Source: CAD feature listing. Evaluate the final solid. Frame: model axes, mm. Coordinates: 2 decimals unless noted, no trailing zeros. Write item = value, one per line. Start each with the question number.
1. Line query: line 1 along X through (y, z) = (21, -3.65); line 2 along X through (y, z) = (0.5, -3.2); line 3 along Y through (x, z) = (-21, -1.2). Output: solid intervals per line, ascending.
2. Section query A-A (x = 29). Give the number of separate pieces and of enclosed holes in the cut face, then the cut area to 3 significant figures.
3. Pin query (flat end, axial travel): pin 1 Ø1.5 at (x, y) = (9, -19.5) entering from +Z; pin 2 Ø1.5 at (x, z) = (0, -2) entering from -Y; pin 3 Ø1.5 at (y, z) = (-13, -2.5) entering from -X; pin 4 Ø1 at (y, z) = (-14.5, -1.5) entering from +X. Return the tip coordinate at first contact, or that it passes through.
```python
from build123d import *

# Parameters (mm, degrees)
F2_DEPTH = 5.08
F3_DEPTH = 5.08


with BuildPart() as f2:
    # F1 (on Top) → F2 (new body)
    with BuildSketch(Plane.XY):
        with BuildLine():
            add(Edge.make_bspline(
                [(-40.3796768019, 31.486727974), (-25.4125832668, 19.5130531459), (4.2719382832, -4.2719382832), (-19.5130531459, 25.4125832668), (-31.486727974, 40.3796768019)],
                knots=[0, 0, 0, 0, 0.5, 1, 1, 1, 1], degree=3))
            Line((-40.3796768019, 31.486727974), (-43.9717792504, 27.8946255256))
            add(Edge.make_bspline(
                [(-43.9717792504, 27.8946255256), (-39.0223614388, 18.5744758569), (-29.1485977035, -0.0186111101), (-39.1966306531, -18.3497362141), (-44.207889928, -27.4920251734)],
                knots=[0, 0, 0, 0, 0.5012696216, 1, 1, 1, 1], degree=3))
            Line((-44.207889928, -27.4920251734), (-40.688852268, -31.1557355805))
            add(Edge.make_bspline(
                [(-40.688852268, -31.1557355805), (-25.5161789229, -19.5156604784), (3.9712190003, 4.6498080898), (-18.7967685048, -26.1767940312), (-30.6525350904, -41.1896309485)],
                knots=[0, 0, 0, 0, 0.4995827747, 1, 1, 1, 1], degree=3))
            Line((-30.6525350904, -41.1896309485), (-26.9813712251, -44.7008922424))
            add(Edge.make_bspline(
                [(-26.9813712251, -44.7008922424), (-17.9946084514, -39.4329857114), (-0.010494669, -28.8909659837), (18.0580501184, -39.3550908644), (27.0976414843, -44.5902337071)],
                knots=[0, 0, 0, 0, 0.4997056226, 1, 1, 1, 1], degree=3))
            Line((27.0976414843, -44.5902337071), (30.7701121053, -41.0803391876))
            add(Edge.make_bspline(
                [(30.7701121053, -41.0803391876), (18.791953604, -26.107641061), (-4.1552313798, 4.3732948199), (25.8949419877, -19.0260044621), (40.8564309314, -30.995195617)],
                knots=[0, 0, 0, 0, 0.5001872305, 1, 1, 1, 1], degree=3))
            Line((40.8564309314, -30.995195617), (44.3699422534, -27.3261850978))
            add(Edge.make_bspline(
                [(44.5902337071, 27.0976414843), (39.403270189, 18.0788208761), (29.0172364099, 0.0201290891), (39.2483982347, -18.2036660263), (44.3699422534, -27.3261850978)],
                knots=[0, 0, 0, 0, 0.4994171624, 1, 1, 1, 1], degree=3))
            Line((44.5902337071, 27.0976414843), (41.0803391876, 30.7701121053))
            add(Edge.make_bspline(
                [(30.995195617, 40.8564309314), (19.0260044621, 25.8949419877), (-4.3732948199, -4.1552313798), (26.107641061, 18.791953604), (41.0803391876, 30.7701121053)],
                knots=[0, 0, 0, 0, 0.4998127695, 1, 1, 1, 1], degree=3))
            Line((30.995195617, 40.8564309314), (27.3261850978, 44.3699422534))
            add(Edge.make_bspline(
                [(-27.8946255256, 43.9717792504), (-18.5644448783, 39.0204369591), (0.0328141053, 29.1512395247), (18.2489978621, 39.3085295686), (27.3261850978, 44.3699422534)],
                knots=[0, 0, 0, 0, 0.5016965487, 1, 1, 1, 1], degree=3))
            Line((-27.8946255256, 43.9717792504), (-31.486727974, 40.3796768019))
        make_face()
    extrude(amount=-F2_DEPTH)

    # F0 (on Top) → F3 (cut, through all)
    with BuildSketch(Plane.XY):
        with BuildLine():
            ThreePointArc((0, -6.35), (4.4901280605, -4.4901280605), (6.35, 0))
            ThreePointArc((6.35, 0), (4.4901280605, 4.4901280605), (0, 6.35))
            ThreePointArc((0, 6.35), (-4.4901280605, 4.4901280605), (-6.35, 0))
            ThreePointArc((-6.35, 0), (-4.4901280605, -4.4901280605), (0, -6.35))
        make_face()
    extrude(amount=-F3_DEPTH, mode=Mode.SUBTRACT)


solid = f2.part
```
Results are:
q1.line_1 = -40.38 to -27.18, -16.24 to 15.59, 28.6 to 41.14
q1.line_2 = -34.13 to -6.33, 6.33 to 34.18
q1.line_3 = -41.25 to -28.69, -16 to 16.24, 27.18 to 40.39
q2.separate_pieces = 3
q2.enclosed_holes = 0
q2.area = 260 mm^2
q3.pin_1 = 0
q3.pin_2 = -34.16
q3.pin_3 = -37.3
q3.pin_4 = 37.92
